Can you work these out from the drawing? Everything is in mm from the part's minimum corner. Give positions to 0.01 mm unless a question says otherwise; leave off trailing zeros. Order: outer loops, then holes, each group sorted by start corner. A loop starts at its lowest first (then second) coordinate and runs counter-clockwise, first axis right, second up. Notation, with made-up numbers: (55, 84.25) -> (111, 84.25) arc R28 cw to (111, 103.25) -> close; hole circle Ø11 at (-32, 56.5). An arc over 180 degrees is marked (long way). Answer as CSV lines item,"result". Start each with the question number.
(1) Will these pins go through, and if not, where does the flat tip stop? pin 1 Ø1.5 at (x, z) = (11.5, 12.5) entering from +Y; pin 2 Ø8 at (x, y) = (29.5, 19) entering from +Z; pin 3 Ø1.5 at (y, z) = (3, 7.5) entering from -X.
(2) I need wall thicknesses on L1, parallel to Z at x = 43, y = 11; L2, parallel to Y at x = 3, z = 17.5; L3, parallel to X at y = 20, z = 13.75 (1 decimal). Which ranges of each line are inside material? Lowest first, please.
(3) I want a section at A-A (x = 7). Please give me the cut outline in (y, z), plus the area to 3 significant figures.
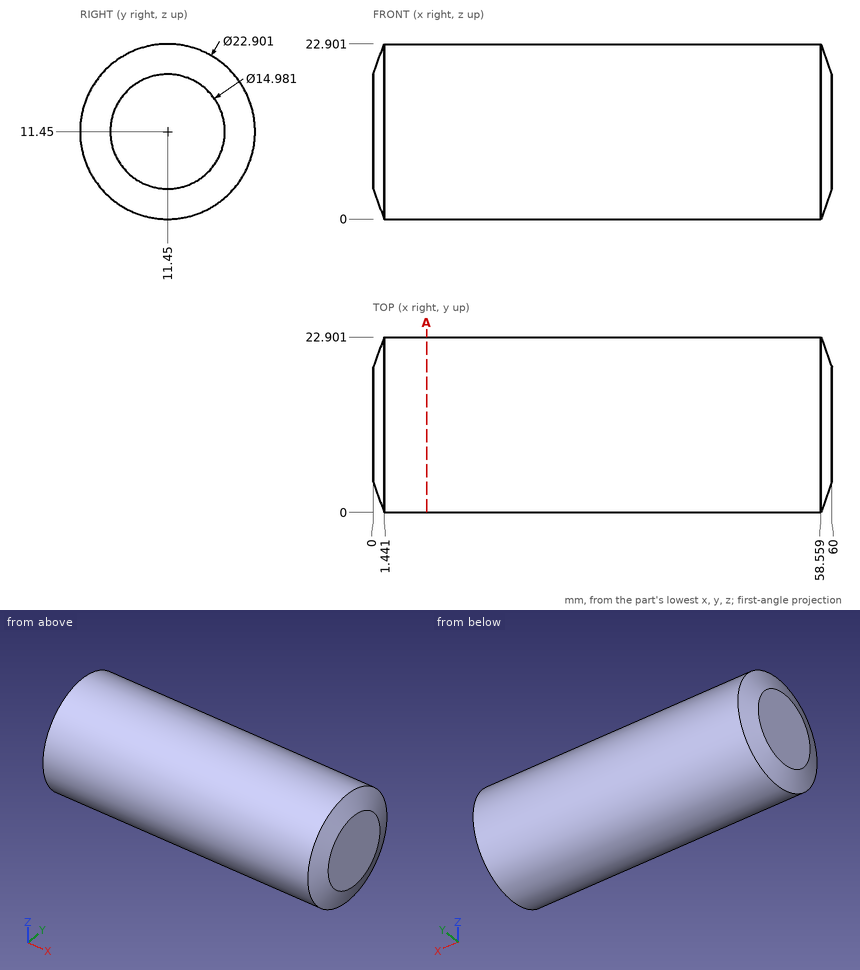
Final values:
1,pin 1,"y = 22.9"
1,pin 2,"z = 22.34"
1,pin 3,"x = 0.4"
2,L1,"0.01 to 22.89"
2,L2,"1.73 to 21.17"
2,L3,"0.5 to 59.5"
3,outline,"circle Ø22.9 at (11.45, 11.45)"
3,area,"412 mm²"
